```python
from build123d import *

# Parameters (mm, degrees)
F0_W     = 48
F0_H     = 55
F1_DEPTH = 15
F2_R     = 17
F3_DEPTH = 30.001
F4_W     = 8
F4_H     = 16
F5_REACH = 72.88954382
F6_R     = 5
F7_REACH = 69.1431356237
F8_W     = 14
F8_H     = 15
F9_DEPTH = 48.001


# Not quite as in the source:
# - a pattern or mirror of a feature is missing from the dataset's text; its kind, count and spacing are read off the source's solid


with BuildPart() as f1:
    # F0 (on Right) → F1 (new body, symmetric)
    with BuildSketch(Plane.YZ):
        Rectangle(F0_W, F0_H)
    extrude(amount=F1_DEPTH, both=True)

    # F2 (on face) → F3 (cut, through all)
    with BuildSketch(Plane.YZ.offset(15)):
        with Locations((0, -1.5)):
            Circle(F2_R)
    extrude(amount=-F3_DEPTH, mode=Mode.SUBTRACT)

    f5_end = f1.faces().sort_by_distance((0, -17, -1.5))[0]
    # F4 (on face) → F5 (cut, up to a face of the model that its end follows)
    with BuildSketch(Plane.XY.offset(27.5)):
        with Locations((11, 0)):
            Rectangle(F4_W, F4_H)
    f5_long = extrude(amount=-F5_REACH, mode=Mode.PRIVATE)
    f5 = split(f5_long, bisect_by=f5_end, keep=Keep.ALL, mode=Mode.PRIVATE).solids().sort_by_distance((11, 0, 27.5))[0]
    add(f5, mode=Mode.SUBTRACT)

    # F5_copies: F5 across plane
    add(f5.mirror(Plane(origin=(0, 0, 0), x_dir=(0, 0, -1), z_dir=(-1, 0, 0))), mode=Mode.SUBTRACT)

    f7_end = f1.faces().sort_by_distance((0, -17, -1.5))[0]
    # F6 (on face) → F7 (cut, up to a face of the model that its end follows)
    with BuildSketch(Plane.XY.offset(27.5)):
        Circle(F6_R)
    f7_long = extrude(amount=-F7_REACH, mode=Mode.PRIVATE)
    add(split(f7_long, bisect_by=f7_end, keep=Keep.ALL, mode=Mode.PRIVATE).solids().sort_by_distance((0, 0, 27.5))[0], mode=Mode.SUBTRACT)

    # F8 (on face) → F9 (cut, through all)
    with BuildSketch(Plane.XZ.offset(24)):
        with Locations((0, -20)):
            Rectangle(F8_W, F8_H)
    extrude(amount=-F9_DEPTH, mode=Mode.SUBTRACT)


solid = f1.part
```
Source: CAD feature listing. Evaluate the final solid. Frame: model axes, mm. A direction names the side the tool comes from. Give positions to 0.01 mm unless a question says otherwise; leave off trailing zeros. Loops run counter-clockwise (first coordinate to the right, second up) from the corner with the lowest first, then second, coordinate; pieces in that order, holes last. Notation, with made-up numbers: (9, -12) -> (43, -12) arc R24 ccw to (43, 21) -> close; hole circle Ø6 at (30, 21). An arc over 180 degrees is marked (long way). Use a Markdown table: item, result. Add a question column.
(1) Section query D-D (z = -16.5). Output: boundary loops of the cut face in (x, y), then the cut area to 3 significant figures.
(2) Section query B-B (y = 0). Output: boundary loops of the cut face in (x, z).
(3) Access query for faces 5 (the face through (7, 0, 21)), 6 (the face through (0, -19, -12.5)), 7 (the face through (-7, 0, 21)), 8 (the face through (0, -6, 27.5)), 9 (the face through (0, -24, 6)). Directions: +Z, -Z, +X, -X, +Y, -Y. A direction counts if a zero-diameter tool reaches every point of the face in a straight line with its end or side. Return the directions, or none.
(4) Section query A-A (z = -1.5). Output: boundary loops of the cut face in (x, y), then the cut area to 3 significant figures.
(5) First-contact query: pin 1 Ø5.5 at (x, y) = (3, -20) entering from -Z; pin 2 Ø1.5 at (x, y) = (-5.5, -2.5) entering from -Z; pin 3 Ø6 at (x, z) = (1.5, -21) entering from -Y; pin 4 Ø6 at (y, z) = (1.5, 14.5) entering from +X. Flat tips, straight axial feed; report the tip coordinate or a pass-through.
(6) Ray query, line 1 (X direction, y = 0, z = 23.5); line 2 (Y direction, x = 3.5, z = -1.5); line 3 (Y direction, x = 8, z = -13). Return the intervals inside material, ascending.
(7) Pull-direction query (X, two-part tool) for faces 1 (the face through (-15, 10, 13)), 2 (the face through (-1.08, -4.88, 21.21)), 3 (the face through (11, -8, 21)), 4 (the face through (0, 18, -12.5)); classes: +X half, -X half, draft (parallel to the pull), parting line (faces both ways), or undercut.
(8) Section query C-C (x = 0). Output: boundary loops of the cut face in (y, z).
Checked values:
| question | item | result |
|---|---|---|
| 1 | outline | (-15, -24) -> (-7, -24) -> (-7, -8) -> (-15, -8) -> close; (-15, 8) -> (-7, 8) -> (-7, 24) -> (-15, 24) -> close; (7, -24) -> (15, -24) -> (15, -8) -> (7, -8) -> close; (7, 8) -> (15, 8) -> (15, 24) -> (7, 24) -> close |
| 1 | area | 512 mm^2 |
| 2 | outline | (-15, -27.5) -> (-7, -27.5) -> (-7, -18.5) -> (-15, -18.5) -> close; (-7, 15.5) -> (-5, 15.5) -> (-5, 27.5) -> (-7, 27.5) -> close; (5, 15.5) -> (7, 15.5) -> (7, 27.5) -> (5, 27.5) -> close; (7, -27.5) -> (15, -27.5) -> (15, -18.5) -> (7, -18.5) -> close |
| 3 | face 5 | +Z, +X |
| 3 | face 6 | -Z, +Y, -Y |
| 3 | face 7 | +Z, -X |
| 3 | face 8 | +Z, +X, -X, +Y, -Y |
| 3 | face 9 | +Z, -Z, +X, -X, -Y |
| 4 | outline | (-15, -24) -> (15, -24) -> (15, -17) -> (-15, -17) -> close; (-15, 17) -> (15, 17) -> (15, 24) -> (-15, 24) -> close |
| 4 | area | 420 mm^2 |
| 5 | pin 1 | z = -12.5 |
| 5 | pin 2 | z = 15.19 |
| 5 | pin 3 | through |
| 5 | pin 4 | x = 7 |
| 6 | line 1 | -7 to -5, 5 to 7 |
| 6 | line 2 | -24 to -17, 17 to 24 |
| 6 | line 3 | -24 to -12.52, 12.52 to 24 |
| 7 | face 1 | -X half |
| 7 | face 2 | undercut |
| 7 | face 3 | draft |
| 7 | face 4 | undercut |
| 8 | outline | (-24, -12.5) -> (-12.96, -12.5) arc R17 cw to (-5, 14.75) -> (-5, 27.5) -> (-24, 27.5) -> close; (5, 14.75) arc R17 cw to (12.96, -12.5) -> (24, -12.5) -> (24, 27.5) -> (5, 27.5) -> close |
